from build123d import *

# Parameters (mm, degrees)
SKETCH1_R           = 8.85
BOSS_EXTRUDE1_DEPTH = 1.25
SKETCH2_R           = 3.45
BOSS_EXTRUDE2_DEPTH = 3.9
SKETCH3_R           = 2
BOSS_EXTRUDE3_DEPTH = 5.6
SKETCH4_W           = 2.828427124
SKETCH4_H           = 2.828427124
BOSS_EXTRUDE4_DEPTH = 2
BOSS_EXTRUDE5_DEPTH = 1.25


with BuildPart() as part:
    # Sketch1 → Boss-Extrude1 (new body)
    with BuildSketch(Plane(origin=(0, 0, 0), x_dir=(1, 0, 0), z_dir=(0, 1, 0))):
        with Locations(Location((0, 0, 0), (0, 0, 270))):
            Circle(SKETCH1_R)
    extrude(amount=BOSS_EXTRUDE1_DEPTH)

    # Sketch2 → Boss-Extrude2 (add)
    with BuildSketch(Plane(origin=(0, 1.25, 0), x_dir=(1, 0, 0), z_dir=(0, 1, 0))):
        with Locations(Location((0, 0, 0), (0, 0, 270))):
            Circle(SKETCH2_R)
    extrude(amount=BOSS_EXTRUDE2_DEPTH)

    # Sketch3 → Boss-Extrude3 (add)
    with BuildSketch(Plane(origin=(0, 5.15, 0), x_dir=(1, 0, 0), z_dir=(0, 1, 0))):
        with Locations(Location((0, 0, 0), (0, 0, 270))):
            Circle(SKETCH3_R)
    extrude(amount=BOSS_EXTRUDE3_DEPTH)

    # Sketch4 → Boss-Extrude4 (add)
    with BuildSketch(Plane(origin=(0, 10.75, 0), x_dir=(1, 0, 0), z_dir=(0, 1, 0))):
        Rectangle(SKETCH4_W, SKETCH4_H)
    extrude(amount=BOSS_EXTRUDE4_DEPTH)

    # Sketch5 → Boss-Extrude5 (add)
    with BuildSketch(Plane.XZ):
        with BuildLine():
            ThreePointArc((-2.65, 8.443932733), (-1.340465463, 8.747894166), (0, 8.85))
            Line((0, 8.85), (0, 13.243932733))
            Line((0, 13.243932733), (-2.4, 13.243932733))
            Line((-2.4, 13.243932733), (-2.65, 8.443932733))
        make_face()
        with BuildLine():
            Line((0, 13.243932733), (0, 8.85))
            ThreePointArc((0, 8.85), (1.340465463, 8.747894166), (2.65, 8.443932733))
            Line((2.65, 8.443932733), (2.4, 13.243932733))
            Line((2.4, 13.243932733), (0, 13.243932733))
        make_face()
    extrude(amount=-BOSS_EXTRUDE5_DEPTH)


solid = part.part
Source: CAD feature listing. Evaluate the final solid. Frame: model axes, mm. A direction names the side the tool comes from. Give positions to 0.01 mm unless a question says otherwise; leave off trailing zeros. Loops run counter-clockwise (first coordinate to the right, second up) from the corner with the lowest first, then second, coordinate; pieces in that order, holes last. Notation, with made-up numbers: (14.25, 2.5) -> (29.25, 2.5) arc R9 ccw to (29.25, 19.5) -> close; hole circle Ø10 at (-18.75, 26.25). An arc over 180 degrees is marked (long way). Use a Markdown table: item, result. Add a question column.
1) First-contact query: pin 1 (5 mm diameter, centred on x = 2, y = 9.5, fed in from +Z); pin 2 (1.5 mm diameter, centred on x = 4, z = -2.5, fed in from +Y); pin 3 (0.6 mm diameter, centred on x = 0.5, z = -2, fed in from +Y). Flat tips, straight axial feed; report the tip coordinate or a pass-through.
2) Section query D-D, the plane y = 3.5. Return the cut outline in (x, z), then the cut area to 3 significant figures.
3) Reachability of faces 1 (the face through (1.414, 12, 0)), 2 (the face through (-1.414, 12, 0)), 3 (the face through (-2, 8, 0)) from +Z, -Z, +X, -X, +Y, -Y: full face, straight path, thin tool, end or side. Return the list, or none.
4) Section query B-B, the plane z = 0. Return the cut outline in (x, y).
5) Section query C-C, the plane y = 6.75. Return the cut outline in (x, z), then the cut area to 3 significant figures.
6) Section query A-A, the plane x = 0. Return the cut outline in (y, z), then the cut area to 3 significant figures.
7) Line query: line 1 along Y through (x, z) = (-7, -0.25); line 2 along Y through (x, z) = (0, 3); line 3 along X through (y, z) = (2.5, 1). Output: solid intervals per line, ascending. Write a range as [from, to].
Numbers:
| question | item | result |
|---|---|---|
| 1 | pin 1 | stops at z = 2 |
| 1 | pin 2 | stops at y = 1.25 |
| 1 | pin 3 | stops at y = 10.75 |
| 2 | outline | circle Ø6.9 at (0, 0) |
| 2 | area | 37.4 mm2 |
| 3 | face 1 | +Z, -Z, +X, +Y |
| 3 | face 2 | +Z, -Z, -X, +Y |
| 3 | face 3 | +Y |
| 4 | outline | (-8.85, 0) -> (8.85, 0) -> (8.85, 1.25) -> (3.45, 1.25) -> (3.45, 5.15) -> (2, 5.15) -> (2, 10.75) -> (1.41, 10.75) -> (1.41, 12.75) -> (-1.41, 12.75) -> (-1.41, 10.75) -> (-2, 10.75) -> (-2, 5.15) -> (-3.45, 5.15) -> (-3.45, 1.25) -> (-8.85, 1.25) -> close |
| 5 | outline | circle Ø4 at (0, 0) |
| 5 | area | 12.6 mm2 |
| 6 | outline | (0, -8.85) -> (1.25, -8.85) -> (1.25, -3.45) -> (5.15, -3.45) -> (5.15, -2) -> (10.75, -2) -> (10.75, -1.41) -> (12.75, -1.41) -> (12.75, 1.41) -> (10.75, 1.41) -> (10.75, 2) -> (5.15, 2) -> (5.15, 3.45) -> (1.25, 3.45) -> (1.25, 13.24) -> (0, 13.24) -> close |
| 6 | area | 82.6 mm2 |
| 7 | line 1 | y = [0, 1.25] |
| 7 | line 2 | y = [0, 5.15] |
| 7 | line 3 | x = [-3.3, 3.3] |
